from build123d import *

# Parameters (mm, degrees)
SALIENTE_EXTRUIR1_DEPTH = 45
CROQUIS3_R              = 19
CORTAR_EXTRUIR1_DEPTH   = 5.6
CROQUIS4_R              = 19
CORTAR_EXTRUIR2_DEPTH   = 5.6
CROQUIS5_W              = 21.8
CROQUIS5_H              = 150
CORTAR_EXTRUIR3_DEPTH   = 55.6
CROQUIS6_W              = 30
CROQUIS6_H              = 10
SALIENTE_EXTRUIR2_DEPTH = 33.6
CROQUIS8_W              = 54.4
CROQUIS8_H              = 19.8
CORTAR_EXTRUIR4_DEPTH   = 1.1
CROQUIS9_W              = 40
CROQUIS9_H              = 19.8
CORTAR_EXTRUIR5_DEPTH   = 22
CROQUIS10_R             = 1.4
CORTAR_EXTRUIR6_DEPTH   = 9
CROQUIS11_W             = 54.4
CROQUIS11_H             = 1.5
CORTAR_EXTRUIR7_DEPTH   = 1.5
CROQUIS12_R             = 8.1
CORTAR_EXTRUIR8_DEPTH   = 17.5
CROQUIS13_R             = 17.5
CORTAR_EXTRUIR9_DEPTH   = 5
CROQUIS14_R             = 1.4
CORTAR_EXTRUIR10_DEPTH  = 5
CROQUIS15_R             = 1.4
CORTAR_EXTRUIR11_DEPTH  = 55
CORTAR_EXTRUIR12_DEPTH  = 2.3
CORTAR_EXTRUIR13_DEPTH  = 2.3
REDONDEO1_R             = 2
REDONDEO1_2_R           = 3


with BuildPart() as part:
    # Croquis2 → Saliente-Extruir1 (new body)
    with BuildSketch(Plane(origin=(0, 0, 0), x_dir=(0, 0, -1), z_dir=(1, 0, 0))):
        with BuildLine():
            Line((0, 25), (100, 25))
            ThreePointArc((100, 25), (125, -1.672e-06), (99.999996656, -25))
            Line((99.999996656, -25), (0, -25))
            ThreePointArc((0, -25), (-25, 0), (0, 25))
        make_face()
    extrude(amount=SALIENTE_EXTRUIR1_DEPTH)

    # Croquis3 → Cortar-Extruir1 (cut)
    with BuildSketch(Plane(origin=(45, 0, 0), x_dir=(0, 0, -1), z_dir=(1, 0, 0))):
        Circle(CROQUIS3_R)
    extrude(amount=-CORTAR_EXTRUIR1_DEPTH, mode=Mode.SUBTRACT)

    # Croquis4 → Cortar-Extruir2 (cut)
    with BuildSketch(Plane.ZY):
        with Locations(Location((0, 0, 0), (0, 0, 180))):  # turned: the seam where the file's is
            Circle(CROQUIS4_R)
    extrude(amount=-CORTAR_EXTRUIR2_DEPTH, mode=Mode.SUBTRACT)

    # Croquis5 → Cortar-Extruir3 (cut)
    with BuildSketch(Plane(origin=(0, 25, 0), x_dir=(1, 0, 0), z_dir=(0, 1, 0))):
        with Locations((22.5, 50)):
            Rectangle(CROQUIS5_W, CROQUIS5_H)
    extrude(amount=-CORTAR_EXTRUIR3_DEPTH, mode=Mode.SUBTRACT)

    # Croquis6 → Saliente-Extruir2 (add)
    with BuildSketch(Plane.ZY.offset(-5.6)):
        with Locations((-50, -1.672e-06)):
            Rectangle(CROQUIS6_W, CROQUIS6_H)
    extrude(amount=-SALIENTE_EXTRUIR2_DEPTH)

    # Croquis8 → Cortar-Extruir4 (cut)
    with BuildSketch(Plane(origin=(45, 0, 0), x_dir=(0, 0, -1), z_dir=(1, 0, 0))):
        with Locations((89.799996656, 0)):
            Rectangle(CROQUIS8_W, CROQUIS8_H)
    extrude(amount=-CORTAR_EXTRUIR4_DEPTH, mode=Mode.SUBTRACT)

    # Croquis9 → Cortar-Extruir5 (cut)
    with BuildSketch(Plane(origin=(43.9, 0, 0), x_dir=(0, 0, -1), z_dir=(1, 0, 0))):
        with Locations((89.799996656, 0)):
            Rectangle(CROQUIS9_W, CROQUIS9_H)
    extrude(amount=-CORTAR_EXTRUIR5_DEPTH, mode=Mode.SUBTRACT)

    # Croquis10 → Cortar-Extruir6 (cut)
    with BuildSketch(Plane(origin=(43.9, 0, 0), x_dir=(0, 0, -1), z_dir=(1, 0, 0))):
        with Locations((65.599996656, -5)):
            Circle(CROQUIS10_R)
        with Locations((65.599996656, 5)):
            Circle(CROQUIS10_R)
        with Locations((113.999996656, 5)):
            Circle(CROQUIS10_R)
        with Locations((113.999996656, -5)):
            Circle(CROQUIS10_R)
    extrude(amount=-CORTAR_EXTRUIR6_DEPTH, mode=Mode.SUBTRACT)

    # Croquis11 → Cortar-Extruir7 (cut)
    with BuildSketch(Plane(origin=(43.9, 0, 0), x_dir=(0, 0, -1), z_dir=(1, 0, 0))):
        with Locations((89.799996656, 0)):
            Rectangle(CROQUIS11_W, CROQUIS11_H)
    extrude(amount=-CORTAR_EXTRUIR7_DEPTH, mode=Mode.SUBTRACT)

    # Croquis12 → Cortar-Extruir8 (cut)
    with BuildSketch(Plane.ZY):
        with Locations((-100, 0)):
            Circle(CROQUIS12_R)
    extrude(amount=-CORTAR_EXTRUIR8_DEPTH, mode=Mode.SUBTRACT)

    # Croquis13 → Cortar-Extruir9 (cut)
    with BuildSketch(Plane.ZY):
        with Locations((-100, 0)):
            Circle(CROQUIS13_R)
    extrude(amount=-CORTAR_EXTRUIR9_DEPTH, mode=Mode.SUBTRACT)

    # Croquis14 → Cortar-Extruir10 (cut)
    with BuildSketch(Plane.ZY.offset(-5)):
        with Locations((-112.8, 0)):
            Circle(CROQUIS14_R)
        with Locations((-87.2, 0)):
            Circle(CROQUIS14_R)
    extrude(amount=-CORTAR_EXTRUIR10_DEPTH, mode=Mode.SUBTRACT)

    # Croquis15 → Cortar-Extruir11 (cut)
    with BuildSketch(Plane.ZY):
        with Locations(Location((-10.3, 0, 0), (0, 0, 180))):  # turned: the seam where the file's is
            Circle(CROQUIS15_R)
        with Locations(Location((10.3, 0, 0), (0, 0, 180))):  # turned: the seam where the file's is
            Circle(CROQUIS15_R)
        with Locations(Location((0, -10.3, 0), (0, 0, 180))):  # turned: the seam where the file's is
            Circle(CROQUIS15_R)
        with Locations(Location((0, 10.3, 0), (0, 0, 180))):  # turned: the seam where the file's is
            Circle(CROQUIS15_R)
    extrude(amount=-CORTAR_EXTRUIR11_DEPTH, mode=Mode.SUBTRACT)

    # Croquis16 → Cortar-Extruir12 (cut)
    with BuildSketch(Plane(origin=(11.6, 0, 0), x_dir=(0, 0, -1), z_dir=(1, 0, 0))):
        Polygon((-7.124573519, 0), (-8.71228676, 2.75), (-11.88771324, 2.75), (-13.475426481, 0), (-11.88771324, -2.75), (-8.71228676, -2.75), align=None)
        Polygon((13.475426481, 0), (11.88771324, 2.75), (8.71228676, 2.75), (7.124573519, 0), (8.71228676, -2.75), (11.88771324, -2.75), align=None)
        Polygon((3.175426481, 10.3), (1.58771324, 13.05), (-1.58771324, 13.05), (-3.175426481, 10.3), (-1.58771324, 7.55), (1.58771324, 7.55), align=None)
        Polygon((3.175426481, -10.3), (1.58771324, -7.55), (-1.58771324, -7.55), (-3.175426481, -10.3), (-1.58771324, -13.05), (1.58771324, -13.05), align=None)
    extrude(amount=-CORTAR_EXTRUIR12_DEPTH, mode=Mode.SUBTRACT)

    # Croquis17 → Cortar-Extruir13 (cut)
    with BuildSketch(Plane.ZY.offset(-33.4)):
        Polygon((3.175426481, 10.3), (1.58771324, 7.55), (-1.58771324, 7.55), (-3.175426481, 10.3), (-1.58771324, 13.05), (1.58771324, 13.05), align=None)
        Polygon((8.71228676, -2.75), (7.124573519, 0), (8.71228676, 2.75), (11.88771324, 2.75), (13.475426481, 0), (11.88771324, -2.75), align=None)
        Polygon((1.58771324, -7.55), (3.175426481, -10.3), (1.58771324, -13.05), (-1.58771324, -13.05), (-3.175426481, -10.3), (-1.58771324, -7.55), align=None)
        Polygon((-7.124573519, 0), (-8.71228676, -2.75), (-11.88771324, -2.75), (-13.475426481, 0), (-11.88771324, 2.75), (-8.71228676, 2.75), align=None)
    extrude(amount=-CORTAR_EXTRUIR13_DEPTH, mode=Mode.SUBTRACT)

    # Redondeo1
    redondeo1_edges = [part.edges().sort_by_distance(p)[0] for p in [
        (45, 25, -50),
        (0, 25, -50),
        (33.4, 25, -50),
        (11.6, 25, -50),
        (22.5, 4.999998328, -65),
        (22.5, -5.000001672, -65),
        (22.5, -5.000001672, -35),
    ]]
    fillet(redondeo1_edges, radius=REDONDEO1_R)

    # Redondeo1 2
    redondeo1_2_edges = [part.edges().sort_by_distance(p)[0] for p in [
        (22.5, 4.999998328, -35),
    ]]
    fillet(redondeo1_2_edges, radius=REDONDEO1_2_R)


solid = part.part
Read the model definition and answer for the solid it produces. Units are mm, in the model's axes. A direction names the side the tool comes from. Give positions to 0.01 mm unless a question says otherwise; leave off trailing zeros. Write each loop counter-clockwise with the first axis right and the second up, starting at its lowest first coordinate (ties: lowest second). Pieces come first, ordered by that corner, then holes. Notation, with made-up numbers: M -4.75,-5.5 L 15.25,-5.5 A21 ccw 15.25,15.5 Z; hole C 40,22 d6. An arc over 180 degrees is marked long. One line per item, written item: value. Start each with the question number.
(1) A tool of negligible diameter and unlimited length cuts with its end or side. For faces 1 (the flat face through (39, 0, -69.8)), 2 (the flat face through (10, 0, -113)), 3 (the flat face through (22, -5, -50)), 4 (the flat face through (9.3, 12, -1)), from which of +Z, -Z, +X, -X, +Y, -Y can it reach the whole face along a straight path? Write none if from no direction.
(2) Flat-ended cylindrical pins translate along their axes: pin 1 Ø4.5 at (y, z) = (-10.3, 0) entering from -X; pin 2 Ø0.8 at (x, y) = (43.5, -4) entering from -Z; pin 3 Ø12 at (x, y) = (38.5, -10.5) entering from -Z. Find the tip coordinate at first contact, or state that the pin passes through.
(3) Find the intervals of material crossed by line 1 (X direction, y = 14.5, z = -77); line 2 (Y direction, x = 10, z = 3); line 3 (X direction, y = 11, z = 3), in increasing order.
(4) Find section C-C (x = 20). Determine the outline of the cut face in (y, z).
(5) Find section B-B (z = -78). Determine the outline of the cut face in (x, y), plus the area to 3 significant figures.
(6) Find section A-A (z = -24.5). Determine the outline of the cut face in (x, y), plus the area to 3 significant figures.
(7) Determine the mould class of faces 5 (the flat face through (43.9, 5.4, -112.5)), 6 (the flat face through (9.3, 1, -12)), 7 (the cylindrical face through (39, 5, -67)) for opening direction X: pulls with the +X half, pulls with the -X half, needs draft (parallel to the pull), parting line crosses it, or undercut.
Results below:
1. face 1: +X
1. face 2: -X
1. face 3: +Z, -Z, -Y
1. face 4: none
2. pin 1: stops at x = 5.6
2. pin 2: stops at z = -124.71
2. pin 3: stops at z = -124.59
3. line 1: x = 0 to 11.6, 33.4 to 45
3. line 2: y = -24.78 to -10.6, -10 to 10, 10.6 to 24.78
3. line 3: x = 5.6 to 11.6, 33.4 to 39.4
4. outline: M -5,-63 A2 ccw -3,-65 L 3,-65 A2 ccw 5,-63 L 5,-38 A3 ccw 2,-35 L -3,-35 A2 ccw -5,-37 Z
5. outline: M 0,-23 A2 ccw 2,-25 L 9.6,-25 A2 ccw 11.6,-23 L 11.6,23 A2 ccw 9.6,25 L 2,25 A2 ccw 0,23 Z; M 33.4,-23 A2 ccw 35.4,-25 L 43,-25 A2 ccw 45,-23 L 45,-9.9 L 33.4,-9.9 Z; M 33.4,9.9 L 45,9.9 L 45,23 A2 ccw 43,25 L 35.4,25 A2 ccw 33.4,23 Z
5. area: 923 mm^2
6. outline: M 0,-23 A2 ccw 2,-25 L 9.6,-25 A2 ccw 11.6,-23 L 11.6,23 A2 ccw 9.6,25 L 2,25 A2 ccw 0,23 Z; M 33.4,-23 A2 ccw 35.4,-25 L 43,-25 A2 ccw 45,-23 L 45,23 A2 ccw 43,25 L 35.4,25 A2 ccw 33.4,23 Z
6. area: 1,150 mm^2
7. face 5: pulls with the +X half
7. face 6: undercut
7. face 7: needs draft
